Part print with two shaded views. Sizes in mm from the minimum x, y, z corner. Round coordinates to 2 decimals unless told otherwise and drop trailing zeros. Order: outer loops, then holes, each group sorted by start corner. A loop starts at its lowest first (then second) coordinate and runs counter-clockwise, first axis right, second up. Notation, with made-up numbers: (13, 17.25) - (51, 17.25) arc R7 cw to (51, 27.25) - close; hole circle Ø2 at (28, 12). An arc over 180 degrees is marked (long way). Use one line per item in the form item = value.
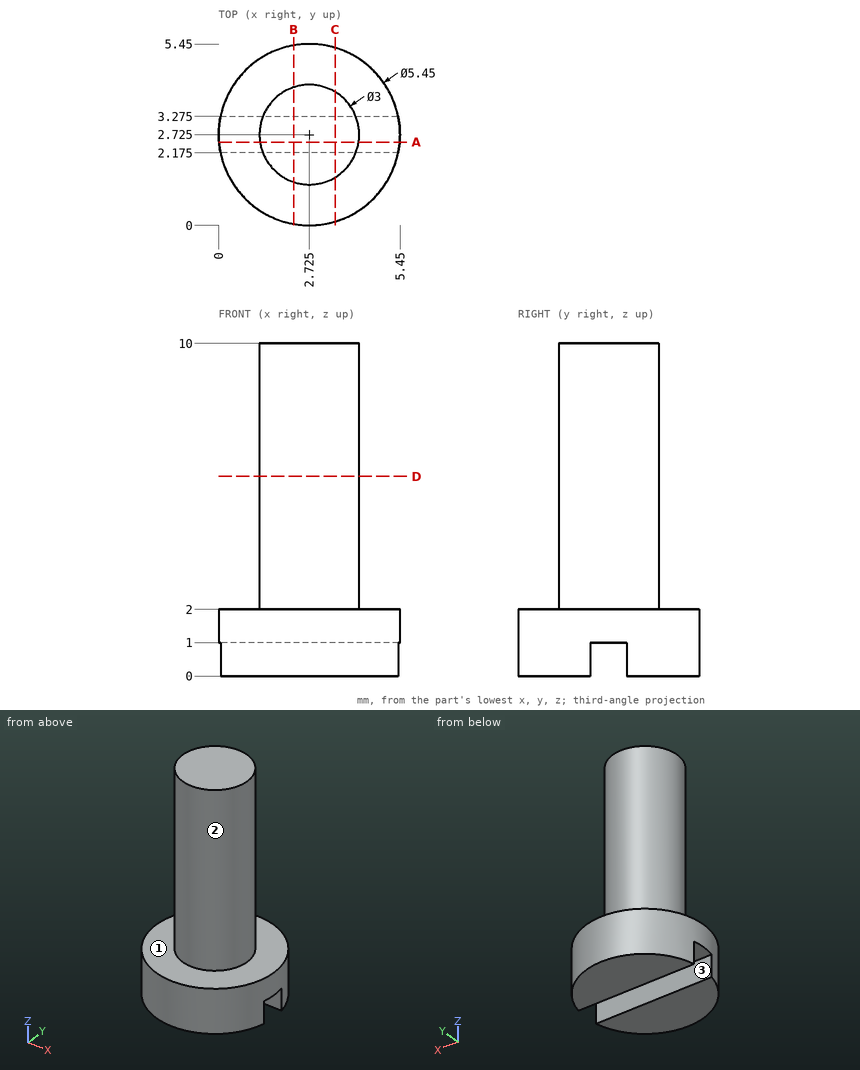
(1) Slice it at A-A on y = 2.5. Give the cut face in (x, z), then the cut area to 3 significant figures.
Report:
outline = (0.01, 1) - (5.44, 1) - (5.44, 2) - (4.21, 2) - (4.21, 10) - (1.24, 10) - (1.24, 2) - (0.01, 2) - close
area = 29.2 mm2
(2) Slice it at D-D on z = 6. Give the cut face in (x, y) (3 decimals).
Report:
outline = circle Ø3 at (2.725, 2.725)
(3) Pin check, flat tips, straight feed: pin 1 (0.8 mm diameter, centred on x = 3.5, z = 0.5, fed in from +Y); pin 2 (1.5 mm diameter, centred on y = 1.5, z = 3.5, fed in from -X); pin 3 (2 mm diameter, centred on x = 1, z = 7.5, fed in from -Y). Stop position of each tip, or through.
Report:
pin_1 = 5.42
pin_2 = 1.3
pin_3 = 1.41
(4) Slice it at C-C on x = 3.5. Give the cut face in (y, z) (3 decimals).
Report:
outline = (0.113, 0) - (2.175, 0) - (2.175, 1) - (3.275, 1) - (3.275, 0) - (5.337, 0) - (5.337, 2) - (4.009, 2) - (4.009, 10) - (1.441, 10) - (1.441, 2) - (0.113, 2) - close
(5) Slice it at B-B on x = 2.25. Give the cut face in (y, z) (3 decimals).
Report:
outline = (0.042, 0) - (2.175, 0) - (2.175, 1) - (3.275, 1) - (3.275, 0) - (5.408, 0) - (5.408, 2) - (4.148, 2) - (4.148, 10) - (1.302, 10) - (1.302, 2) - (0.042, 2) - close
(6) Pull direction Y, two halves, no side cores. Call the marked faces 1, 2 and 3: released by +Y, released by -Y, zero draft, split by the parting line, or undercut.
Report:
face_1 = zero draft
face_2 = split by the parting line
face_3 = undercut
(7) Probe probe 1 along Z at (x, y) = (1.6, 4.85); probe 2 along Y at (x, z) = (2.7, 2.5). List the from-to ranges inside material, lowest first. Write a range as [from, to].
Report:
probe_1 = [0, 2]
probe_2 = [1.23, 4.22]
